Design review of the part built by this model. Coordinates are the model's own, in mm. A direction names the side the tool comes from. Give positions to 0.01 mm unless a question says otherwise; leave off trailing zeros. Write each loop counter-clockwise with the first axis right and the second up, starting at its lowest first coordinate (ties: lowest second). Pieces come first, ordered by that corner, then holes. Notation, with made-up numbers: (-25, 72) -> (-18, 72) arc R17 cw to (-18, 97) -> close; hole circle Ø6 at (36, -6.75). An arc over 180 degrees is marked (long way). Answer as a JSON object with one key per item and string values.
```python
from build123d import *

# Parameters (mm, degrees)
SKIZZE1_W                       = 162
SKIZZE1_H                       = 42
AUFSATZ_LINEAR_AUSTRAGEN1_DEPTH = 33
SKIZZE2_R                       = 8
SCHNITT_LINEAR_AUSTRAGEN1_DEPTH = 28
VERRUNDUNG1_R                   = 3.5
SCHNITT_LINEAR_AUSTRAGEN2_DEPTH = 89.238313821


with BuildPart() as part:
    # Skizze1 → Aufsatz-Linear austragen1 (new body)
    with BuildSketch(Plane(origin=(0, 0, 0), x_dir=(1, 0, 0), z_dir=(0, 1, 0))):
        Rectangle(SKIZZE1_W, SKIZZE1_H)
    extrude(amount=AUFSATZ_LINEAR_AUSTRAGEN1_DEPTH)

    # Skizze2 → Schnitt-Linear austragen1 (cut)
    with BuildSketch(Plane(origin=(0, 33, 0), x_dir=(1, 0, 0), z_dir=(0, 1, 0))):
        with Locations((-81, -21)):
            Circle(SKIZZE2_R)
        with Locations((81, 21)):
            Circle(SKIZZE2_R)
    extrude(amount=-SCHNITT_LINEAR_AUSTRAGEN1_DEPTH, mode=Mode.SUBTRACT)

    # Verrundung1
    verrundung1_edges = [part.edges().sort_by_distance(p)[0] for p in [
        (81, 33, 4),
        (4, 33, 21),
        (-75.343145751, 33, 15.343145751),
        (-4, 33, -21),
        (75.343145751, 33, -15.343145751),
        (-81, 33, -4),
        (-81, 16.5, -21),
        (81, 16.5, 21),
    ]]
    fillet(verrundung1_edges, radius=VERRUNDUNG1_R)

    # Skizze3 → Schnitt-Linear austragen2 (cut, through all)
    with BuildSketch(Plane(origin=(0, 5, 0), x_dir=(1, 0, 0), z_dir=(0, 1, 0))):
        with BuildLine():
            Line((76.262563133, 18.737436867), (79.762563133, 22.237436867))
            ThreePointArc((79.762563133, 22.237436867), (82.237436867, 22.237436867), (82.237436867, 19.762563133))
            Line((82.237436867, 19.762563133), (78.737436867, 16.262563133))
            ThreePointArc((78.737436867, 16.262563133), (76.262563133, 16.262563133), (76.262563133, 18.737436867))
        make_face()
        with BuildLine():
            Line((-76.262563133, -18.737436867), (-79.762563133, -22.237436867))
            ThreePointArc((-79.762563133, -22.237436867), (-82.237436867, -22.237436867), (-82.237436867, -19.762563133))
            Line((-82.237436867, -19.762563133), (-78.737436867, -16.262563133))
            ThreePointArc((-78.737436867, -16.262563133), (-76.262563133, -16.262563133), (-76.262563133, -18.737436867))
        make_face()
    extrude(amount=-SCHNITT_LINEAR_AUSTRAGEN2_DEPTH, mode=Mode.SUBTRACT)


solid = part.part
```
(1) For line 1 along Y through (x, z) = (-59, -19); line 2 along X through (y, z) = (13.5, -15.5); line 3 along X through (y, z) = (30.5, 16), list the stretches that pass through material, from the lowest coordinate up.
Here are the results:
{"line 1": "y = 0 to 32.66", "line 2": "x = -81 to 75.19", "line 3": "x = -74.57 to 80.85"}
(2) Clearance check with flat-ended pins moving along their axes: pin 1 (6.5 mm diameter, centred on x = -77, z = 15.5, fed in from +Y); pin 2 (6.5 mm diameter, centred on x = 75.5, z = -16, fed in from +Y). State where each tip first meets the part, or that it passes through.
Here are the results:
{"pin 1": "stops at y = 32.69", "pin 2": "stops at y = 32.9"}
(3) The part is to be moulded in two halves that separate along Z. For faces 1 (the flat face through (-1, 33, 0)), 2 (the cylindrical face through (75.281, 17.422, -15.406)), 3 (the flat face through (-2, 15, 21)), 4 (the cylindrical face through (76.29, 2.535, -16.236)), say which applies: +Z half, -Z half, draft (parallel to the pull), parting line (faces both ways), or undercut.
Here are the results:
{"face 1": "draft", "face 2": "-Z half", "face 3": "+Z half", "face 4": "undercut"}
(4) We need section A-A, the plane y = 16.5. State the section outline as (x, z) points, then the cut area to 3 significant figures.
Here are the results:
{"outline": "(-81, -17.5) arc R3.5 ccw to (-77.5, -21) -> (73, -21) arc R8 cw to (81, -13) -> (81, 17.5) arc R3.5 ccw to (77.5, 21) -> (-73, 21) arc R8 cw to (-81, 13) -> close", "area": "6,700 mm²"}
(5) For faces 5 (the cylindrical face through (-80, 14.96, -19.95)), 6 (the flat face through (-76, 5, 16)), 7 (the flat face through (76, 5, -16)), list the 3-axis set-ups (+Z, -Z, +X, -X, +Y, -Y) from which the entire face can be reached by the end or side of a thin tool; tool diameter is ignored.
Here are the results:
{"face 5": "-Z, -X, +Y, -Y", "face 6": "+Z, -X, +Y", "face 7": "-Z, +X, +Y"}
